Input: dimensioned drawing with shaded views. Units: mm. Origin: part minimum x, y, z. A direction names the side the tool comes from. Give positions to 0.01 mm unless a question says otherwise; leave off trailing zeros. Loops run counter-clockwise (first coordinate to the right, second up) from the corner with the lowest first, then second, coordinate; pieces in that order, holes last.
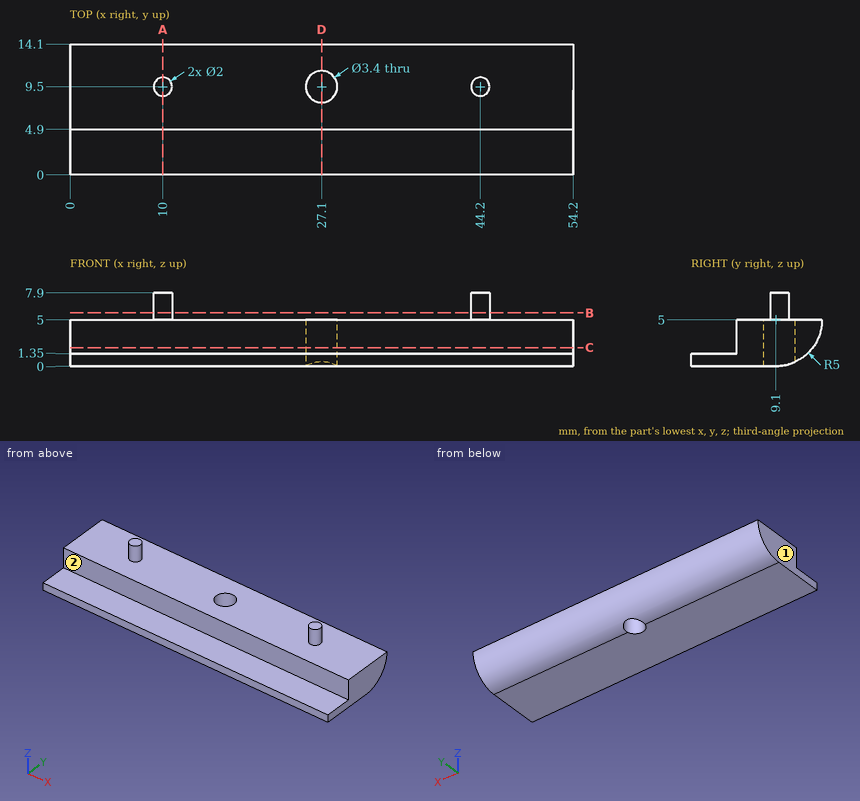
Item 1: Pin query (flat end, axial travel): pin 1 (5 mm diameter, centred on x = 26.5, y = 12, fed in from -Z); pin 2 (4.5 mm diameter, centred on x = 27.1, y = 9.5, fed in from +Z); pin 3 (3 mm diameter, centred on x = 14, z = 3, fed in from +Y); pin 4 (4 mm diameter, centred on x = 19, z = 3, fed in from -Y). Return the tip coordinate at first contact, or that it passes through.
Values follow:
pin 1: stops at z = 0.04
pin 2: stops at z = 5
pin 3: stops at y = 14.07
pin 4: stops at y = 0
Item 2: Section query A-A on x = 10. Return loops of the section in (y, z), plus the area to 4 significant figures.
Values follow:
outline: (0, 0) - (9.1, 0) arc R5 ccw to (14.1, 5) - (10.5, 5) - (10.5, 7.9) - (8.5, 7.9) - (8.5, 5) - (4.9, 5) - (4.9, 1.35) - (0, 1.35) - close
area: 53.05 mm2
Item 3: Section query C-C on z = 2. Return loops of the section in (x, y), plus the area to 3 significant figures.
Values follow:
outline: (0, 4.9) - (54.2, 4.9) - (54.2, 13.1) - (0, 13.1) - close; hole circle Ø3.4 at (27.1, 9.5)
area: 435 mm2
Item 4: Ray query, probe 1 along X at (y, z) = (9.5, 2.5); probe 2 along Z at (x, y) = (31, 2); probe 3 along Y at (x, z) = (27.1, 2.75). Return the intervals inside material, ascending.
Values follow:
probe 1: x = 0 to 25.4, 28.8 to 54.2
probe 2: z = 0 to 1.35
probe 3: y = 4.9 to 7.8, 11.2 to 13.57
Item 5: Section query B-B on z = 5.75. Return loops of the section in (x, y).
Values follow:
outline: circle Ø2 at (10, 9.5); circle Ø2 at (44.2, 9.5)
Item 6: Set-up query: the marked faces 1 and 2. Return all of +Z, -Z, +X, -X, +Y, -Y with unobstructed straight access to the full face (end or side cutting, diameter ignored); none if empty.
Values follow:
face 1: +Z, -Z, -X, +Y, -Y
face 2: +Z, +X, -X, -Y
Item 7: Section query D-D on x = 27.1. Return loops of the section in (y, z).
Values follow:
outline: (0, 0) - (7.8, 0) - (7.8, 5) - (4.9, 5) - (4.9, 1.35) - (0, 1.35) - close; (11.2, 0.46) arc R5 ccw to (14.1, 5) - (11.2, 5) - close
